Here's the drawing with two shaded views (mm, measured from the low corner). I have some questions. Coordinates: 2 decimals unless noted, no trailing zeros. Order: outer loops, then holes, each group sorted by start corner. A loop starts at its lowest first (then second) coordinate and runs counter-clockwise, first axis right, second up. Notation, with made-up numbers: (75, 26.25) -> (80, 26.25) arc R19 cw to (80, 45.25) -> close; hole circle Ø9 at (83, 7.5). An arc over 180 degrees is marked (long way). Return JSON: item names as keys, results as strings. Group by question number.
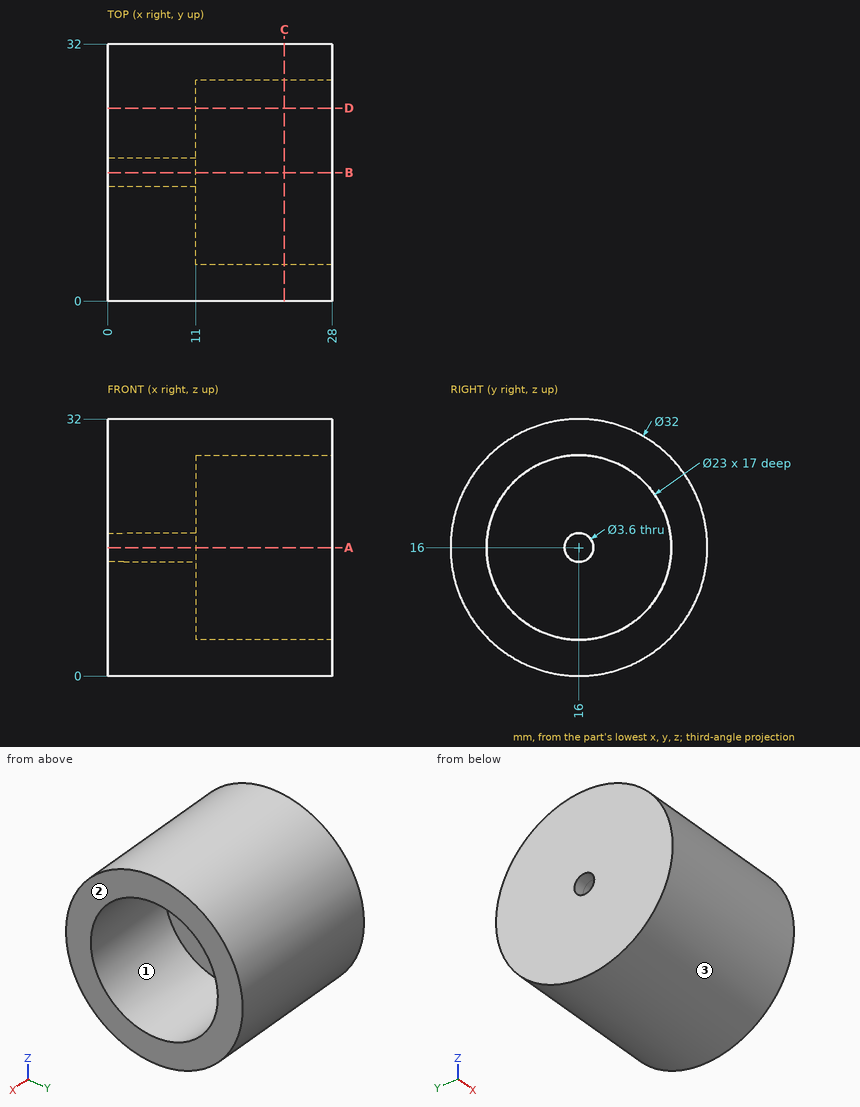
Q1. I need wall thicknesses on line 1 along Z through (x, y) = (7.75, 16); line 2 along Z through (x, y) = (14.75, 16); line 3 along X through (y, z) = (11, 25). Which ranges of each line are inside material? Lowest first, please. Write a range as from..to.
Q2. I want a section at A-A on z = 16. Please give me the cut outline in (x, y).
Q3. I want a section at C-C on x = 22. Please give me the cut outline in (y, z).
Q4. I'm going to push flat-ended pins straight in: pin 1 Ø11.5 at (y, z) = (19, 18) entering from +X; pin 2 Ø6 at (x, z) = (23, 23) entering from -Y; pin 3 Ø10 at (y, z) = (10, 19.5) entering from -X; pin 4 Ø6 at (x, y) = (20.5, 28) entering from -Z. Where does each tip first touch, or does it pass through?
Q5. I want a section at D-D on y = 24. Please give me the cut outline in (x, z).
Q6. We'd pull the mould along Z, two halves only. Please class the marked faces 1, 2 and 3: pulls with the +Z half, pulls with the -Z half, needs draft (parallel to the pull), parting line crosses it, or undercut.
Response values:
{
 "1": {"line 1": "z = 0..14.2, 17.8..32", "line 2": "z = 0..4.5, 27.5..32", "line 3": "x = 0..11"},
 "2": {"outline": "(0, 0) -> (28, 0) -> (28, 4.5) -> (11, 4.5) -> (11, 14.2) -> (0, 14.2) -> close; (0, 17.8) -> (11, 17.8) -> (11, 27.5) -> (28, 27.5) -> (28, 32) -> (0, 32) -> close"},
 "3": {"outline": "circle Ø32 at (16, 16); hole circle Ø23 at (16, 16)"},
 "4": {"pin 1": "stops at x = 11", "pin 2": "stops at y = 0.51", "pin 3": "stops at x = 0", "pin 4": "stops at z = 2.77"},
 "5": {"outline": "(0, 2.14) -> (28, 2.14) -> (28, 7.74) -> (11, 7.74) -> (11, 24.26) -> (28, 24.26) -> (28, 29.86) -> (0, 29.86) -> close"},
 "6": {"face 1": "undercut", "face 2": "needs draft", "face 3": "parting line crosses it"}
}
